Input: part model. Units: mm. Frame: model coordinates. A direction names the side the tool comes from. Give positions to 0.01 mm unless a question says otherwise; leave off trailing zeros. Loops run counter-clockwise (first coordinate to the right, second up) from the corner with the lowest first, then second, coordinate; pieces in that order, holes last. Notation, with made-up numbers: (51, -22.75) - (110, -22.75) arc R28 cw to (110, 16.25) - close; hole circle Ø8 at (-18, 4.5). An arc over 180 degrees is marked (long way). One line per question, with ' | ' between items. Start each with the question number.
from build123d import *

# Parameters (mm, degrees)
F1_DEPTH  = 4
F2_R      = 3.99999
F3_R      = 2.5
F4_DEPTH  = 8
F6_DEPTH  = 4
F9_R      = 4
F10_DEPTH = 6.851053331


# Not quite as in the source:
# - a fillet or chamfer that OpenCascade refuses, or shapes differently, is made with other operations: its cross-section is extruded or revolved along the edge and cut away or added
# - a fillet or chamfer is up to 0.001 mm smaller than in the source, because OpenCascade refuses the exact size


with BuildPart() as f1:
    # F0 (on Front) → F1 (new body, symmetric)
    with BuildSketch(Plane.XZ):
        Polygon((-26.6568542495, 0), (0, 0), (0, 8), (-34.6568542495, 8), align=None)
    extrude(amount=F1_DEPTH, both=True)

    # F2 (radius 4 in the source; OpenCascade refuses exactly that, so slightly less here)
    f2_edges = [f1.edges().sort_by_distance(p)[0] for p in [
        (-30.656854, 4, 4),
        (-30.656854, -4, 4),
    ]]
    fillet(f2_edges, radius=F2_R)

    # F3 (on face) → F4 (cut, through all)
    with BuildSketch(Plane.XY.offset(8)):
        with Locations((-14.5, 0)):
            Circle(F3_R)
    extrude(amount=-F4_DEPTH, mode=Mode.SUBTRACT)

    # F5 (on face) → F6 (cut)
    with BuildSketch(Plane.XY.offset(8)):
        with BuildLine():
            ThreePointArc((-14.5, 4), (-10.5, 0), (-14.5, -4))
            Line((-14.5, -4), (0, -4))
            Line((0, -4), (0, 4))
            Line((0, 4), (-14.5, 4))
        make_face()
    extrude(amount=-F6_DEPTH, mode=Mode.SUBTRACT)

    # F9 (on line) → F10 (join, symmetric)
    with BuildSketch(Plane(origin=(-18.5, 0, 18.5), x_dir=(0, 1, 0), z_dir=(0.7071067812, 0, -0.7071067812))):
        with Locations((0, -14.8492424049)):
            Circle(F9_R)
    extrude(amount=F10_DEPTH, both=True)

    # F7 (on Front) → F11 (revolve, cut)
    with BuildSketch(Plane.XZ):
        Polygon((-20.5108239612, -2.6104963823), (-19.4501637894, -1.5498362106), (-43.5361095251, 22.5361095251), (-44.5967696969, 21.4754493533), align=None)
    revolve(axis=Axis((-31.4931366573, 0, 10.4931366573), (-0.7071067812, 0, 0.7071067812)), mode=Mode.SUBTRACT)

    # F12: chamfer of 1 x 3.7320508076 on 1 edges, made by hand

    # F12_s1 → F12_t2 (revolve, cut)
    with BuildSketch(Plane(origin=(-10.5, 0, -10.5), x_dir=(0, 1, 0), z_dir=(-0.7071067812, 0, -0.7071067812))):
        Polygon((4, -29.2819534274), (3, -33.0140042349), (4, -33.0140042349), align=None)
    revolve(axis=Axis((-33.8444262687, 0, 12.8444262687), (0.7071067812, 0, -0.7071067812)), mode=Mode.SUBTRACT)

    # F13: F1 across face


with BuildPart() as f1_1:
    add(f1.part)
    add(f1.part.mirror(Plane(origin=(0, 0, 2), x_dir=(0, 1, 0), z_dir=(1, 0, 0))))


solid = f1_1.part
Q1. Section A-A, the plane x = 9. Output: boundary loops of the cut face in (y, z), plus the area to 3 significant figures.
Q2. First-contact query: pin 1 (2.5 mm diameter, centred on x = 17, y = -1.5, fed in from +Z); pin 2 (2 mm diameter, centred on x = 15.5, y = -0.5, fed in from +Z) (3 decimals); pin 3 (2 mm diameter, centred on y = -2.5, z = 4, fed in from +X); pin 4 (2.5 mm diameter, centred on x = -3.5, y = 2, fed in from +Z). Flat tips, straight axial feed; report the tip coordinate or a pass-through.
Q3. Access query for faces 4 (the face through (0, 0, 0)), 5 (the face through (-10.5, 0.1, 6)). Directions: +Z, -Z, +X, -X, +Y, -Y. A direction counts if a zero-diameter tool reaches every point of the face in a straight line with its end or side. Return the directions, or none.
Q4. Line query: L1, parallel to Y at x = 14.5, z = 4.5; L2, parallel to X at y = 1, z = 8.5; L3, parallel to X at y = 1, z = 7.75. Output: solid intervals per line, ascending. Write a range as from..to.
Q5. Draft query along X for faces 1 (the face through (34.76, 1.29, 11.93)), 2 (the face through (-25.68, -0.07, 6.8)), 3 (the face through (0, 4, 3)). Return one class per face: +X half, -X half, draft (parallel to the pull), parting line (faces both ways), or undercut.
Q6. Section B-B, the plane z = 5. Count the separate pieces of the cut face and the enclosed holes in it, plus the area to 3 significant figures.
Solved:
1) outline: (-4, 0) - (4, 0) - (4, 4) - (-4, 4) - close | area: 32.0 mm²
2) pin 1: stops at z = 8 | pin 2: passes through | pin 3: stops at x = 30.78 | pin 4: stops at z = 4
3) face 4: -Z, +X, -X, +Y, -Y | face 5: +Z
4) L1: y = -4..-2.5, 2.5..4 | L2: x = -34.53..-31.08, -27.92..-24.02, 24.02..27.92, 31.08..34.53 | L3: x = -34.1..-30.33, -27.17..-16.79, -12.21..-10.63, 10.63..12.21, 16.79..27.17, 30.33..34.1
5) face 1: +X half | face 2: undercut | face 3: draft
6) separate pieces: 2 | enclosed holes: 4 | area: 246 mm²
